Read the model definition and answer for the solid it produces. Units are mm, in the model's axes. Face numbers are marked on the shaded views. A direction names the side the tool comes from. Coordinates: 2 decimals unless noted, no trailing zeros. Loops run counter-clockwise (first coordinate to the right, second up) from the corner with the lowest first, then second, coordinate; pieces in that order, holes last. Notation, with made-up numbers: (-40, -24) - (9, -24) arc R28 cw to (9, 15) - close; hole circle Ø6 at (26.5, -23). An arc over 180 degrees is marked (long way). One line per item, written item: value. Start each with the question number.
from build123d import *

# Parameters (mm, degrees)
F1_DEPTH  = 800
F3_DEPTH  = 2
F5_DEPTH  = 2
F7_DEPTH  = 25
F9_DEPTH  = 25
F11_R     = 15
F12_DEPTH = 10


with BuildPart() as f1:
    # F0 (on Front) → F1 (new body)
    with BuildSketch(Plane.XZ):
        Polygon((-202.4154143159, 327.6886455222), (-204.1763566452, 326.7404461164), (0, -17.224690761), (195.7943682295, 331.5797893846), (194.0503458287, 332.5587612257), (0, -13.1387713996), align=None)
    extrude(amount=F1_DEPTH)

    # F2 (on face) → F3 (join)
    with BuildSketch(Plane.XZ.offset(800)):
        Polygon((0, -13.1387713996), (171.3200722008, 292.0651487278), (-180.4445918465, 286.7607939107), align=None)
    extrude(amount=-F3_DEPTH)

    # F4 (on face) → F5 (join)
    with BuildSketch(Plane(origin=(0, 0, 0), x_dir=(-1, 0, 0), z_dir=(0, 1, 0))):
        Polygon((-171.3200722008, 287.9792293664), (0, -17.224690761), (178.6543120645, 283.7448040067), align=None)
    extrude(amount=F5_DEPTH)

    # F6 (on face) → F7 (join)
    with BuildSketch(Plane(origin=(0, 2, 0), x_dir=(-1, 0, 0), z_dir=(0, 1, 0))):
        Polygon((-67.7318355426, 103.4384718181), (-81.0449193734, 127.1555139717), (-261.7674144737, -108.3666270862), (-230.2556041235, -108.3666270862), align=None)
        Polygon((261.7674144737, -108.3666270862), (83.6715723559, 123.7323931592), (69.9270135898, 100.5776600892), (230.2556041235, -108.3666270862), align=None)
        Polygon((83.6715723559, 123.7323931592), (0, 232.775309239), (-81.0449193734, 127.1555139717), (-67.7318355426, 103.4384718181), (0, 191.7083184464), (69.9270135898, 100.5776600892), align=None)
    extrude(amount=F7_DEPTH)

    # F8 (on face) → F9 (join)
    with BuildSketch(Plane.XZ.offset(800)):
        Polygon((81.0449193734, 127.1555139717), (0, 232.775309239), (-83.6715723559, 123.7323931592), (-69.9270135898, 100.5776600892), (0, 191.7083184464), (67.1786031406, 102.4528972986), align=None)
        Polygon((261.7674144737, -108.3666270862), (81.0449193734, 127.1555139717), (67.1786031406, 102.4528972986), (225.8531237559, -108.3666270862), align=None)
        Polygon((-69.9270135898, 100.5776600892), (-83.6715723559, 123.7323931592), (-261.7674144737, -108.3666270862), (-230.2556041235, -108.3666270862), align=None)
    extrude(amount=F9_DEPTH)

    # F11 (on face) → F12 (cut)
    with BuildSketch(Plane(origin=(-7.5605140907, 0, -4.4878915213), x_dir=(0, -1, 0), z_dir=(-0.8599128422, 0, -0.5104408916))):
        with Locations((400, 82.1180880011)):
            Circle(F11_R)
        with Locations((306.596378018, 82.1180880011)):
            Circle(F11_R)
        with Locations((200, 82.1180880011)):
            Circle(F11_R)
        with Locations((100, 82.1180880011)):
            Circle(F11_R)
        with Locations((500, 82.1180880011)):
            Circle(F11_R)
        with Locations((600, 82.1180880011)):
            Circle(F11_R)
        with Locations((700, 82.1180880011)):
            Circle(F11_R)
    extrude(amount=-F12_DEPTH, mode=Mode.SUBTRACT)


solid = f1.part
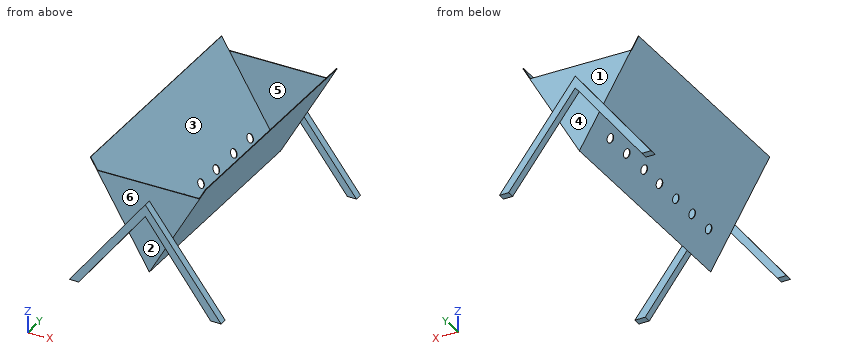
1) Flat-ended cylindrical pins translate along their axes: P1, Ø10, axis at x = -16, y = -683.5, coming from the +Z side; P2, Ø4, axis at x = 34.5, y = -260.5, coming from the +Z side; P3, Ø12, axis at y = -659.5, z = 49.5, coming from the -X side. Find the tip coordinate at first contact, or state that the pin passes through.
2) Straight lines are drawn through the part: L1, parallel to Y at x = 52.5, z = 192; L2, parallel to X at y = -384, z = 114; L3, parallel to X at y = -22.5, z = 231.5. For each, find the intervals that lie inside material, in ascending order.
3) Section A-A, the plane z = 43.5 is taken. Determine the outline of the cut face in (x, y), and give its area (3 significant figures).
4) Section C-C, the plane y = -360 is taken. Determine the outline of the cut face in (x, z), and give its area (3 significant figures).
5) Section D-D, the plane z = -47.5 is taken. Determine the outline of the cut face in (x, y).
6) Section B-B, the plane x = 111 is taken. Determine the outline of the cut face in (y, z), and give its area (3 significant figures).
7) For the marked faces 1 and 2, determine the directions among +Z, -Z, +X, -X, +Y, -Y from which every point of the face is accessible in a straight line to the end or side of a thin tool.
8) Determine the mould class of the marked faces 3, 4, 5 and 6 for opening direction Y: released by +Y, released by -Y, zero draft, split by the parting line, or undercut.
Answer below:
1. P1: z = 22.22
1. P2: z = 51.89
1. P3: x = -43.17
2. L1: -800 to -798, 0 to 2
2. L2: -77.89 to -75.51, 71.37 to 73.66
2. L3: -147.64 to -145.29, 137.32 to 139.62
3. outline: (-145.24, -825) - (-113.72, -825) - (-113.72, -800) - (-145.24, -800) - close; (-145.24, 2) - (-113.72, 2) - (-113.72, 27) - (-145.24, 27) - close; (-36.05, -800) - (34.09, -800) - (34.09, 2) - (-36.05, 2) - close; (111.55, -825) - (145.24, -825) - (145.24, -800) - (111.55, -800) - close; (113.72, 2) - (145.24, 2) - (145.24, 27) - (113.72, 27) - close; hole (-33.64, -798) - (31.79, -798) - (31.79, 0) - (-33.64, 0) - close
3. area: 7,240 mm2
4. outline: (-204.18, 326.74) - (0, -17.22) - (195.79, 331.58) - (194.05, 332.56) - (0, -13.14) - (-202.42, 327.69) - close
4. area: 1,610 mm2
5. outline: (-215.06, -825) - (-183.55, -825) - (-183.55, -800) - (-215.06, -800) - close; (-215.06, 2) - (-183.55, 2) - (-183.55, 27) - (-215.06, 27) - close; (180.04, -825) - (215.06, -825) - (215.06, -800) - (180.04, -800) - close; (183.55, 2) - (215.06, 2) - (215.06, 27) - (183.55, 27) - close
6. outline: (-825, 44.23) - (-800, 44.23) - (-800, 88.12) - (-825, 88.12) - close; (-800, 180.52) - (2, 180.52) - (2, 287.25) - (0, 287.25) - (0, 184.61) - (-798, 184.61) - (-798, 291.16) - (-800, 291.16) - close; (2, 47.05) - (27, 47.05) - (27, 88.12) - (2, 88.12) - close
6. area: 5,820 mm2
7. face 1: +Z, +Y
7. face 2: -Z, -Y
8. face 3: undercut
8. face 4: released by +Y
8. face 5: undercut
8. face 6: released by -Y
